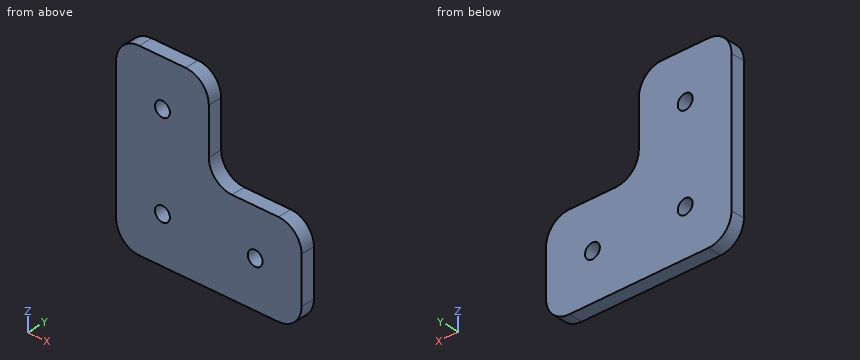
```python
from build123d import *

# Parameters (mm, degrees)
SKETCH_1_R      = 1.6
EXTRUDE_1_DEPTH = 3
FILLET_1_R      = 5


with BuildPart() as part:
    # 草图1 → 凸台-拉伸1 (new body)
    with BuildSketch(Plane(origin=(0, 0, 0), x_dir=(1, 0, 0), z_dir=(0, 1, 0))):
        Polygon((0, 0), (0, 40), (40, 40), (40, 20), (20, 20), (20, 0), align=None)
        with Locations(Location((30, 30, 0), (0, 0, 270))):
            Circle(SKETCH_1_R, mode=Mode.SUBTRACT)
        with Locations(Location((10, 30, 0), (0, 0, 270))):
            Circle(SKETCH_1_R, mode=Mode.SUBTRACT)
        with Locations(Location((10, 10, 0), (0, 0, 270))):
            Circle(SKETCH_1_R, mode=Mode.SUBTRACT)
    extrude(amount=EXTRUDE_1_DEPTH)

    # 圆角1
    fillet_1_edges = [part.edges().sort_by_distance(p)[0] for p in [
        (0, 1.5, 0),
        (0, 1.5, -40),
        (40, 1.5, -40),
        (40, 1.5, -20),
        (20, 1.5, -20),
        (20, 1.5, 0),
    ]]
    fillet(fillet_1_edges, radius=FILLET_1_R)


solid = part.part
```
Geometry: final body of the model. Coordinates: model frame, mm. Coordinates: 2 decimals unless noted, no trailing zeros. Loops run counter-clockwise (first coordinate to the right, second up) from the corner with the lowest first, then second, coordinate; pieces in that order, holes last. Notation, with made-up numbers: (-18.5, 46) -> (-7.5, 46) arc R12 ccw to (-7.5, 55) -> close; hole circle Ø8 at (24.5, 63). An arc over 180 degrees is marked (long way). Use a Markdown table: item, result. Add a question column.
(1) Section query C-C, the plane z = -30. Return loops of the section in (x, y).
(2) Section query D-D, the plane x = 30. Return loops of the section in (y, z).
(3) Section query A-A, the plane y = 0.9. Return loops of the section in (x, z), plus the area to 3 significant figures.
(4) Line query: line 1 along X through (y, z) = (1.15, -30); line 2 along X through (y, z) = (0.9, -10); line 3 along X through (y, z) = (2.85, -31). Output: solid intervals per line, ascending.
(5) Section query B-B, the plane x = 10. Return loops of the section in (y, z), plus the area to 3 significant figures.
Answer:
| question | item | result |
|---|---|---|
| 1 | outline | (0, 0) -> (8.4, 0) -> (8.4, 3) -> (0, 3) -> close; (11.6, 0) -> (28.4, 0) -> (28.4, 3) -> (11.6, 3) -> close; (31.6, 0) -> (40, 0) -> (40, 3) -> (31.6, 3) -> close |
| 2 | outline | (0, -40) -> (3, -40) -> (3, -31.6) -> (0, -31.6) -> close; (0, -28.4) -> (3, -28.4) -> (3, -20) -> (0, -20) -> close |
| 3 | outline | (0, -35) arc R5 ccw to (5, -40) -> (35, -40) arc R5 ccw to (40, -35) -> (40, -25) arc R5 ccw to (35, -20) -> (25, -20) arc R5 cw to (20, -15) -> (20, -5) arc R5 ccw to (15, 0) -> (5, 0) arc R5 ccw to (0, -5) -> close; hole circle Ø3.2 at (10, -30); hole circle Ø3.2 at (10, -10); hole circle Ø3.2 at (30, -30) |
| 3 | area | 1,150 mm^2 |
| 4 | line 1 | x = 0 to 8.4, 11.6 to 28.4, 31.6 to 40 |
| 4 | line 2 | x = 0 to 8.4, 11.6 to 20 |
| 4 | line 3 | x = 0 to 8.75, 11.25 to 28.75, 31.25 to 40 |
| 5 | outline | (0, -40) -> (3, -40) -> (3, -31.6) -> (0, -31.6) -> close; (0, -28.4) -> (3, -28.4) -> (3, -11.6) -> (0, -11.6) -> close; (0, -8.4) -> (3, -8.4) -> (3, 0) -> (0, 0) -> close |
| 5 | area | 101 mm^2 |
